Autodesk Inventor part; units mm, degrees
ref_plane "YZ Plane" through (0, 0, 0) normal (1, 0, 0) x (0, 1, 0)
ref_plane "XZ Plane" through (0, 0, 0) normal (0, 1, 0) x (-1, 0, 0)
ref_plane "XY Plane" through (0, 0, 0) normal (0, 0, 1) x (1, 0, 0)
sketch "スケッチ1" plane through (0, 0, 0) normal (0, 1, 0) x (-1, 0, 0)
  line L0 (-8, 10) -> (8, 10)
  line L1 (8, 10) -> (8, -10)
  line L2 (8, -10) -> (-8, -10)
  line L3 (-8, -10) -> (-8, 10)
  line L4 (-8, 10) -> (8, -10) construction
  line L5 (8, 10) -> (-8, -10) construction
  circle A0 centre (0, 15) radius 5
  circle A1 centre (0, -15) radius 5
  line L6 (4.4944, 17.191) -> (8, 10)
  line L7 (-8, 10) -> (-4.4944, 17.191)
  line L8 (4.4944, -17.191) -> (8, -10)
  line L9 (-8, -10) -> (-4.4944, -17.191)
  point P0 (0, 0)
  dimension "d0" = 16
  dimension "d1" = 20
  dimension "d2" = 10
  dimension "d3" = 10
extrude "押し出し1" add sketch "スケッチ1" along normal blind 2
sketch "スケッチ4" plane through (0, 2, 0) normal (0, 1, 0) x (1, 0, 0)
  arc A0 (-4.4944, -17.191) -> (4.4944, -17.191) centre (0, -15) ccw
  arc A1 (4.4944, 17.191) -> (-4.4944, 17.191) centre (0, 15) ccw
  point P0 (0, 0)
hole "穴1" at (0, 2, 15) at (0, 2, -15) direction (0, -1, 0) diameter 3.5 end through all
fillet "フィレット1" radius 2 4 edges at (8, 1, 10) (8, 1, -10) (-8, 1, -10) (-8, 1, 10)
sketch "スケッチ5" plane through (0, 2, 0) normal (0, 1, 0) x (1, 0, 0)
  line L0 (8, -9.5385) -> (8, 9.5385)
  line L1 (-8, -6.5) -> (8, -6.5)
  line L2 (8, -6.5) -> (8, 6.5)
  line L3 (8, 6.5) -> (-8, 6.5)
  line L4 (-8, 6.5) -> (-8, -6.5)
  line L5 (-8, -6.5) -> (8, 6.5) construction
  line L6 (8, -6.5) -> (-8, 6.5) construction
  line L7 (-2.4, -6.5) -> (2.4, -6.5)
  line L8 (2.4, -6.5) -> (2.4, 6.5)
  line L9 (2.4, 6.5) -> (-2.4, 6.5)
  line L10 (-2.4, 6.5) -> (-2.4, -6.5)
  line L11 (-2.4, -6.5) -> (2.4, 6.5) construction
  line L12 (2.4, -6.5) -> (-2.4, 6.5) construction
  line L13 (-8, 9.5385) -> (-8, -9.5385)
  line L14 (5.25, -6.5) -> (-5.25, -6.5)
  line L15 (-5.25, -6.5) -> (-5.25, 6.5)
  line L16 (-5.25, 6.5) -> (5.25, 6.5)
  line L17 (5.25, 6.5) -> (5.25, -6.5)
  line L18 (5.25, -6.5) -> (-5.25, 6.5) construction
  line L19 (-5.25, -6.5) -> (5.25, 6.5) construction
  point P0 (0, 0)
  dimension "d28" = 13
  dimension "d29" = 4.8
  dimension "d33" = 10.5
extrude "押し出し4" cut sketch "スケッチ5" against normal through all contours L1 L8 L3 L17 | L1 L15 L3 L10
fillet "フィレット2" radius 0.4 8 edges at (-2.4, 1, 6.5) (2.4, 1, 6.5) (2.4, 1, -6.5) (-2.4, 1, -6.5) (-5.25, 1, 6.5) (-5.25, 1, -6.5) (5.25, 1, -6.5) (5.25, 1, 6.5)
equation "\"d3\" = d2"
properties part number "3D_bno055_bottom_3D プリント"
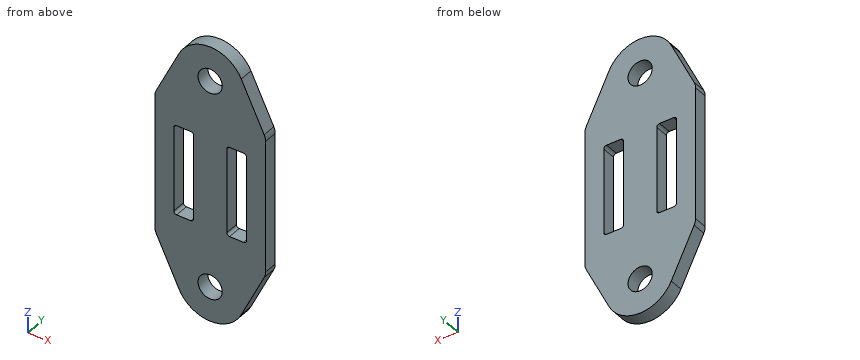
Input: part model. Units: mm. Frame: model coordinates. Round coordinates to 2 decimals unless told otherwise and drop trailing zeros. Loops run counter-clockwise (first coordinate to the right, second up) from the corner with the lowest first, then second, coordinate; pieces in that order, holes last. Notation, with made-up numbers: M 28,26 L 48,26 A19 cw 48,63 Z; hole C 88,78.5 d3. An arc over 180 degrees is marked long. Answer as CSV lines item,"result". Start each with the question number.
(1) Line query: line 1 (Z direction, x = 0, y = 1.4); line 2 (X direction, y = 1.75, z = -3); line 3 (X direction, y = 0.45, z = -15). Output: solid intervals per line, ascending. Write a range as [from, to].
(2) Section A-A, the plane z = 0. Output: boundary loops of the cut face in (x, y), plus the area to 3 significant figures.
(3) Section B-B, the plane x = 0. Output: boundary loops of the cut face in (y, z), plus the area to 3 significant figures.
(4) Section C-C, the plane z = -15. Output: boundary loops of the cut face in (x, y).
(5) First-contact query: pin 1 (0.6 mm diameter, centred on x = -3.5, y = 1.5, fed in from +Z); pin 2 (1 mm diameter, centred on x = 3.5, y = 1, fed in from -Z); pin 3 (0.6 mm diameter, centred on x = 4, y = 1.5, fed in from +Z). Flat tips, straight axial feed; report the tip coordinate or a pass-through.
(6) Section D-D, the plane y = 0.35. State how many separate pieces and enclosed holes the cut face has, plus the area to 3 significant figures.
Values found:
1,line 1,"z = [-20, -16.75], [-13.25, 13.25], [16.75, 20]"
1,line 2,"x = [-8, -5.25], [-2.4, 2.4], [5.25, 8]"
1,line 3,"x = [-5.56, -1.75], [1.75, 5.56]"
2,outline,"M -8,0 L -5.25,0 L -5.25,2 L -8,2 Z; M -2.4,0 L 2.4,0 L 2.4,2 L -2.4,2 Z; M 5.25,0 L 8,0 L 8,2 L 5.25,2 Z"
2,area,"20.6 mm²"
3,outline,"M 0,-20 L 2,-20 L 2,-16.75 L 0,-16.75 Z; M 0,-13.25 L 2,-13.25 L 2,13.25 L 0,13.25 Z; M 0,16.75 L 2,16.75 L 2,20 L 0,20 Z"
3,area,"66.0 mm²"
4,outline,"M -5.56,0 L -1.75,0 L -1.75,2 L -5.56,2 Z; M 1.75,0 L 5.56,0 L 5.56,2 L 1.75,2 Z"
5,pin 1,"stops at z = 18.84"
5,pin 2,"stops at z = -19"
5,pin 3,"stops at z = 18.36"
6,separate pieces,"1"
6,enclosed holes,"4"
6,area,"443 mm²"
